Geometry: final body of the model. Coordinates: model frame, mm. A direction names the side the tool comes from. Give positions to 0.01 mm unless a question says otherwise; leave off trailing zeros. Order: outer loops, then holes, each group sorted by start corner. A loop starts at its lowest first (then second) coordinate and runs counter-clockwise, first axis right, second up. Notation, with made-up numbers: (-11.5, 62.25) - (9.5, 62.25) arc R11 ccw to (9.5, 83.25) - close; hole circle Ø5 at (61.25, 2). An arc over 180 degrees is marked (long way). One line per item, written item: value.
```python
from build123d import *

# Parameters (mm, degrees)
BOSS_EXTRUDE2_DEPTH = 2
SKETCH9_R           = 2
CUT_EXTRUDE1_DEPTH  = 10


with BuildPart() as part:
    # Sketch1 → Revolve1 (revolve)
    with BuildSketch(Plane.XY):
        Polygon((-4.5, 0), (-1.5, 0), (-1.5, -3.5), (-2.5, -3.5), (-2.5, -2.5), (-4.25, -2.5), (-4.5, -2.25), align=None)
        Polygon((0.5, -2.75), (4.25, -2.75), (4.5, -2.5), (4.5, 0), (0.5, 0), align=None)
    revolve(axis=Axis((-4.5, 0, 0), (1, 0, 0)))

    # Sketch5 → Boss-Extrude2 (add)
    with BuildSketch(Plane(origin=(-1.5, 0, 0), x_dir=(0, 0, -1), z_dir=(1, 0, 0))):
        Polygon((1.911716384, -4.204601503), (4.597149907, -0.446705798), (2.685433523, 3.757895705), (-1.911716384, 4.204601503), (-4.597149907, 0.446705798), (-2.685433523, -3.757895705), align=None)
    extrude(amount=BOSS_EXTRUDE2_DEPTH)

    # Sketch9 → Cut-Extrude1 (cut)
    with BuildSketch(Plane(origin=(4.5, 0, 0), x_dir=(0, 0, -1), z_dir=(1, 0, 0))):
        Circle(SKETCH9_R)
    extrude(amount=-CUT_EXTRUDE1_DEPTH, mode=Mode.SUBTRACT)


solid = part.part
```
1) Set-up query: faces 5 (the face through (-2.5, -2, 2)), 6 (the face through (-0.514, -1.626, 3.655)), 7 (the face through (2.401, 0.596, 2.685)). Return all of +Z, -Z, +X, -X, +Y, -Y with unobstructed straight access to the full face (end or side cutting, diameter ignored); none if empty.
Answers below:
face 5: -X
face 6: +Z, +X, -X, -Y
face 7: +X
2) Mould query, pull axis Z, two halves, no side actions, for faces 1 (the face through (0, -2, 0)), 2 (the face through (-3.39, 0.54, 2.44)), 3 (the face through (-0.514, 1.626, -3.655)), 4 (the face through (-0.51, -3.98, 0.42)). Classes: released by +Z, released by -Z, zero draft, split by the parting line, or undercut.
Answers below:
face 1: undercut
face 2: split by the parting line
face 3: released by -Z
face 4: released by +Z
3) First-contact query: pin 1 (2.5 mm diameter, centred on y = -1, z = -1.5, fed in from +X); pin 2 (1.5 mm diameter, centred on x = -1.5, y = 1.5, fed in from +Z); pin 3 (4 mm diameter, centred on x = 1, z = -2, fed in from +Y). Flat tips, straight axial feed; report the tip coordinate or a pass-through.
Answers below:
pin 1: x = 4.5
pin 2: z = 4.38
pin 3: y = 4.01
4) Section D-D, the plane z = -3. Return loops of the section in (x, y).
Answers below:
outline: (-2.5, -1.8) - (-1.5, -1.8) - (-1.5, -2.68) - (0.5, -2.68) - (0.5, 3.07) - (-1.5, 3.07) - (-1.5, 1.8) - (-2.5, 1.8) - close
5) Section C-C, the plane z = 0. Return loops of the section in (x, y), then the cut area to 3 significant figures.
Answers below:
outline: (-4.5, -2.25) - (-4.25, -2.5) - (-2.5, -2.5) - (-2.5, -3.5) - (-1.5, -3.5) - (-1.5, -4.02) - (0.5, -4.02) - (0.5, -2.75) - (4.25, -2.75) - (4.5, -2.5) - (4.5, -2) - (-4.5, -2) - close; (-4.5, 2) - (4.5, 2) - (4.5, 2.5) - (4.25, 2.75) - (0.5, 2.75) - (0.5, 4.02) - (-1.5, 4.02) - (-1.5, 3.5) - (-2.5, 3.5) - (-2.5, 2.5) - (-4.25, 2.5) - (-4.5, 2.25) - close
area: 19.0 mm^2
6) Section B-B, the plane x = 3.5. Return loops of the section in (y, z).
Answers below:
outline: circle Ø5.5 at (0, 0); hole circle Ø4 at (0, 0)
7) Material intervals for line 1 along Y through (x, z) = (-2, 0); line 2 along X through (y, z) = (3.25, 1.75); line 3 along Y through (x, z) = (3, -0.25), sorted ascending.
Answers below:
line 1: -3.5 to -2, 2 to 3.5
line 2: -1.5 to 0.5
line 3: -2.74 to -1.98, 1.98 to 2.74
8) Section A-A, the plane y = 0. Return loops of the section in (x, z), then the cut area to 3 significant figures.
Answers below:
outline: (-4.5, -2.25) - (-4.25, -2.5) - (-2.5, -2.5) - (-2.5, -3.5) - (-1.5, -3.5) - (-1.5, -4.39) - (0.5, -4.39) - (0.5, -2.75) - (4.25, -2.75) - (4.5, -2.5) - (4.5, -2) - (-4.5, -2) - close; (-4.5, 2) - (4.5, 2) - (4.5, 2.5) - (4.25, 2.75) - (0.5, 2.75) - (0.5, 4.39) - (-1.5, 4.39) - (-1.5, 3.5) - (-2.5, 3.5) - (-2.5, 2.5) - (-4.25, 2.5) - (-4.5, 2.25) - close
area: 20.5 mm^2
